The drawing under review shows one solid part. Ordinate dimensions are in mm from its lowest x, y, z. Give positions to 0.01 mm unless a question says otherwise; leave off trailing zeros. Loops run counter-clockwise (first coordinate to the right, second up) from the corner with the lowest first, then second, coordinate; pieces in that order, holes last. Notation, with made-up numbers: (88.25, 57.25) -> (114.25, 57.25) arc R24 ccw to (114.25, 91.25) -> close; hole circle Ø5 at (72.25, 85). An arc over 180 degrees is marked (long way). Answer in a Markdown table with one row per item. Add a question column.
(1) Consider section C-C on y = 6.5. Write out the cut boundary in (x, z).
(2) Draft analysis for pull direction Y (two halves, no side actions). For the marked faces 1 and 2, state which applies: +Y half, -Y half, draft (parallel to the pull), parting line (faces both ways), or undercut.
(3) Consider section D-D on x = 182.5. Write out the cut boundary in (y, z), then the cut area to 3 significant figures.
(4) Consider section B-B on z = 12.5. Write out the cut boundary in (x, y).
(5) For line 1 (X direction, y = 1.25, z = 12.5); line 2 (X direction, y = 1.25, z = 54.5); line 3 (Z direction, x = 24, y = 3.5), list the stretches that pass through material, from the lowest coordinate up.
(6) For pin 1 (5 mm diameter, centred on x = 88, y = 6.5, fed in from -Z); pin 2 (1.8 mm diameter, centred on y = 3.5, z = 55, fed in from -X), all flat-tipped, find the tip position at first contact; note any pin that passes through.
(7) Consider section A-A on x = 32.5. Write out the cut boundary in (y, z), then the cut area to 3 significant figures.
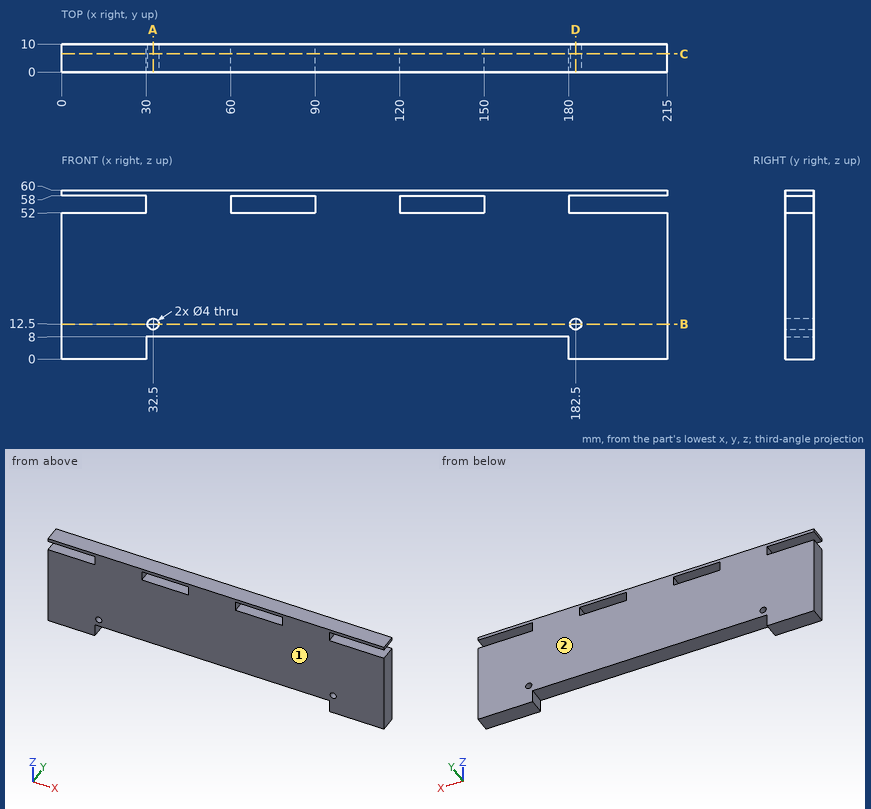
Values follow:
| question | item | result |
|---|---|---|
| 1 | outline | (0, 0) -> (30, 0) -> (30, 8) -> (180, 8) -> (180, 0) -> (215, 0) -> (215, 52) -> (180, 52) -> (180, 58) -> (215, 58) -> (215, 60) -> (0, 60) -> (0, 58) -> (30, 58) -> (30, 52) -> (0, 52) -> close; hole circle Ø4 at (32.5, 12.5); hole (60, 52) -> (90, 52) -> (90, 58) -> (60, 58) -> close; hole (120, 52) -> (150, 52) -> (150, 58) -> (120, 58) -> close; hole circle Ø4 at (182.5, 12.5) |
| 2 | face 1 | -Y half |
| 2 | face 2 | +Y half |
| 3 | outline | (0, 0) -> (10, 0) -> (10, 10.5) -> (0, 10.5) -> close; (0, 14.5) -> (10, 14.5) -> (10, 52) -> (0, 52) -> close; (0, 58) -> (10, 58) -> (10, 60) -> (0, 60) -> close |
| 3 | area | 500 mm2 |
| 4 | outline | (0, 0) -> (30.5, 0) -> (30.5, 10) -> (0, 10) -> close; (34.5, 0) -> (180.5, 0) -> (180.5, 10) -> (34.5, 10) -> close; (184.5, 0) -> (215, 0) -> (215, 10) -> (184.5, 10) -> close |
| 5 | line 1 | 0 to 30.5, 34.5 to 180.5, 184.5 to 215 |
| 5 | line 2 | 30 to 60, 90 to 120, 150 to 180 |
| 5 | line 3 | 0 to 52, 58 to 60 |
| 6 | pin 1 | z = 8 |
| 6 | pin 2 | x = 30 |
| 7 | outline | (0, 8) -> (10, 8) -> (10, 10.5) -> (0, 10.5) -> close; (0, 14.5) -> (10, 14.5) -> (10, 60) -> (0, 60) -> close |
| 7 | area | 480 mm2 |
